Could you check a few things on this drawing? It's one solid part, dimensions in mm from its lowest x, y, z. Give positions to 0.01 mm unless a question says otherwise; leave off trailing zeros. Loops run counter-clockwise (first coordinate to the right, second up) from the corner with the lowest first, then second, coordinate; pieces in that order, holes last. Notation, with made-up numbers: (45.25, 42) - (91.25, 42) arc R23 ccw to (91.25, 76) - close; hole circle Ø6 at (-37, 15.25). An arc over 180 degrees is marked (long way). Use CSV: the item, a comma, the result in double quotes.
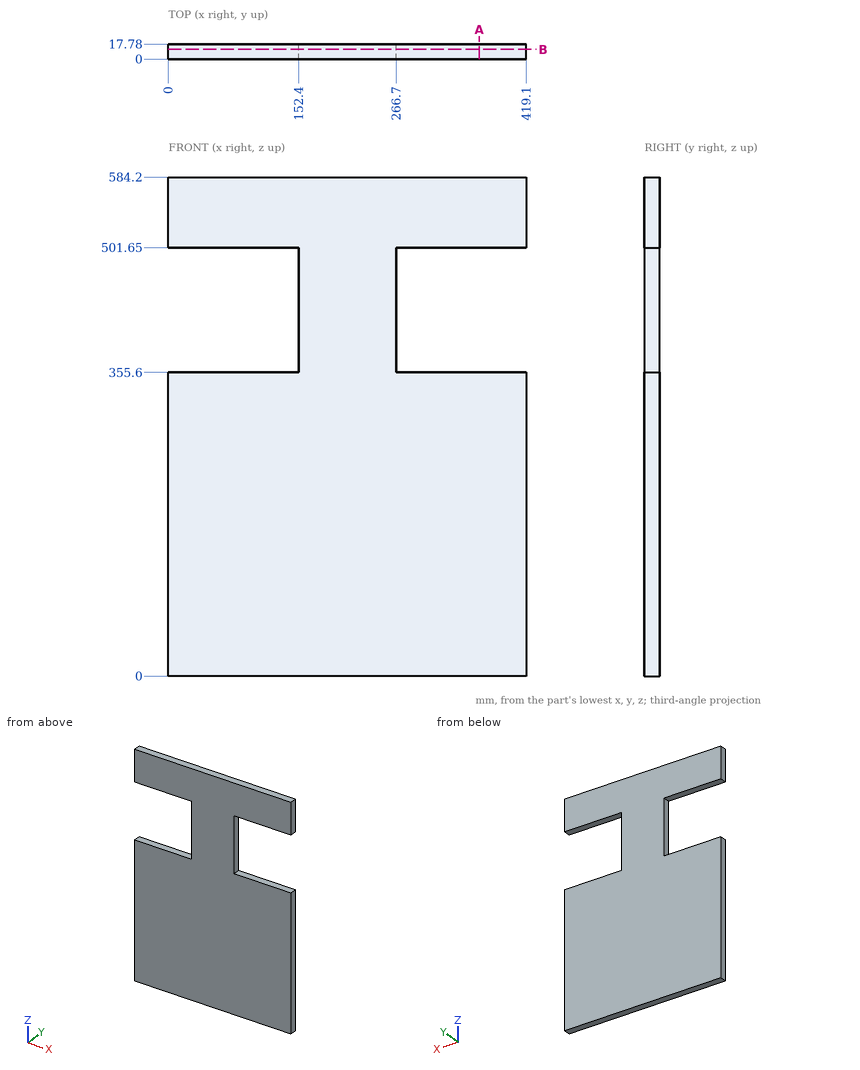
1) Suppose I cut it at B-B (y = 11.5). Please give me the cut outline in (x, z), plus the area to 3 significant figures.
Answer below:
outline,"(0, 0) - (419.1, 0) - (419.1, 355.6) - (266.7, 355.6) - (266.7, 501.65) - (419.1, 501.65) - (419.1, 584.2) - (0, 584.2) - (0, 501.65) - (152.4, 501.65) - (152.4, 355.6) - (0, 355.6) - close"
area,"200,000 mm2"
2) I'm going to push a flat-ended pin straight in: P1, Ø1.5, axis at x = 250.5, z = 511, coming from the -Y side. Where does the tip first touch, or does it pass through?
Answer below:
P1,"stops at y = 0"
3) Suppose I cut it at A-A (x = 364). Please give me the cut outline in (y, z), plus the area to 3 significant figures.
Answer below:
outline,"(0, 0) - (17.78, 0) - (17.78, 355.6) - (0, 355.6) - close; (0, 501.65) - (17.78, 501.65) - (17.78, 584.2) - (0, 584.2) - close"
area,"7,790 mm2"
4) I need wall thicknesses on line 1 along Z through (x, y) = (395, 16.75); line 2 along X through (y, z) = (8.75, 401.5). Which ranges of each line are inside material? Lowest first, please.
Answer below:
line 1,"z = 0 to 355.6, 501.65 to 584.2"
line 2,"x = 152.4 to 266.7"
